For this review, take the finished solid that the model builds, in its own axes (mm). Face numbers are marked on the shaded views. Coordinates: 2 decimals unless noted, no trailing zeros. Write each loop counter-clockwise with the first axis right and the second up, starting at its lowest first coordinate (ties: lowest second). Pieces come first, ordered by that corner, then holes.
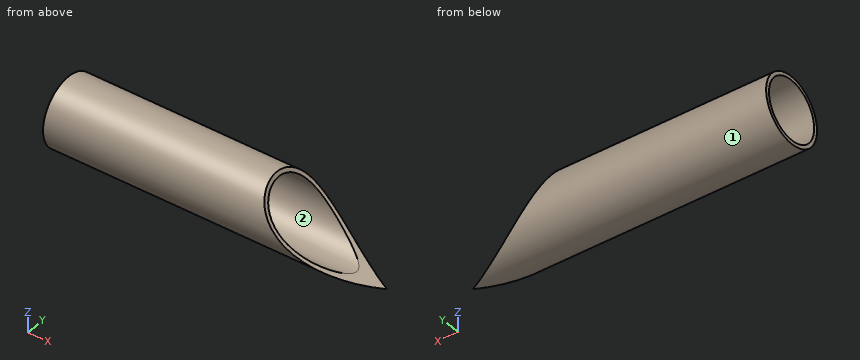
```python
from build123d import *

# Parameters (mm, degrees)
F0_R     = 8.5
F0_R_2   = 7.55
F1_DEPTH = 80
F2_R     = 31
F3_DEPTH = 25.4
F4_DEPTH = 25.4
F6_ANGLE = -90
F8_ANGLE = -90


with BuildPart() as f1:
    # F0 (on Top) → F1 (new body)
    with BuildSketch(Plane.XY):
        Circle(F0_R)
        Circle(F0_R_2, mode=Mode.SUBTRACT)
    extrude(amount=F1_DEPTH)

    # F2 (on Right) → F3 (cut)
    with BuildSketch(Plane.YZ):
        with Locations((22.5, 0)):
            Circle(F2_R)
    extrude(amount=-F3_DEPTH, mode=Mode.SUBTRACT)

    # F2 (on Right) → F4 (cut)
    with BuildSketch(Plane.YZ):
        with Locations((22.5, 0)):
            Circle(F2_R)
    extrude(amount=F4_DEPTH, mode=Mode.SUBTRACT)


with BuildPart() as f1_1:
    # F6: moved
    add(f1.part.rotate(Axis((14.042603, 0, 0), (-1, 0, 0)), F6_ANGLE))


with BuildPart() as f1_2:
    # F8: moved
    add(f1_1.part.rotate(Axis((0, 0, 13.531513), (0, 0, 1)), F8_ANGLE))


solid = f1_2.part
```
1) For L1, parallel to Z at x = -33, y = 0.25; L2, parallel to Y at x = -45.5, z = -6.25; L3, parallel to Y at x = -46, z = -2.75, list the stretches that pass through material, from the lowest coordinate up.
2) The part is to be moulded in two halves that separate along Y. For the marked faces 1 and 2, say which applies: pulls with the +Y half, pulls with the -Y half, needs draft (parallel to the pull), parting line crosses it, or undercut.
3) Consider section B-B (y = -3). Give the boundary of the cut face in (x, z), then the cut area to 3 significant figures.
4) Consider section D-D (x = -13). Give the boundary of the cut face in (y, z).
5) Consider section A-A (z = -6.5). Give the boundary of the cut face in (x, y), then the cut area to 3 significant figures.
6) Consider section C-C (x = -50). Give the boundary of the cut face in (y, z).
7) Clearance check with flat-ended pins moving along their axes: P1, Ø1, axis at x = -49, z = -2.5, coming from the +Y side; P2, Ø6, axis at x = -66.5, z = 1, coming from the -Y side; P3, Ø6, axis at x = -63.5, z = 6, coming from the +Y side; P4, Ø1, axis at x = -65, y = 5, coming from the -Z side. State where each tip first meets the part, or that it passes through.
Results:
1. L1: z = -8.5 to -7.55, 7.55 to 8.5
1. L2: y = -5.76 to -4.24, 4.24 to 5.76
1. L3: y = -8.04 to -7.03, 7.03 to 8.04
2. face 1: parting line crosses it
2. face 2: undercut
3. outline: (-80, -7.95) - (-5.8, -7.95) arc R31 cw to (-9.75, -6.93) - (-80, -6.93) - close; (-80, 6.93) - (-26.81, 6.93) arc R31 cw to (-27.37, 7.95) - (-80, 7.95) - close
3. area: 128 mm2
4. outline: (-6.36, -5.64) arc R8.5 ccw to (6.36, -5.64) - (5.02, -5.64) arc R7.55 cw to (-5.02, -5.64) - close
5. outline: (-80, -5.48) - (-10.95, -5.48) - (-10.95, -3.84) - (-80, -3.84) - close; (-80, 3.84) - (-10.95, 3.84) - (-10.95, 5.48) - (-80, 5.48) - close
5. area: 226 mm2
6. outline: circle Ø17 at (0, 0); hole circle Ø15.1 at (0, 0)
7. P1: stops at y = 8.26
7. P2: stops at y = -8.5
7. P3: stops at y = 7.95
7. P4: stops at z = -7.21
